Geometry check sheet. Reference: drawing and pictorial views, mm from the part's lowest x, y, z. Round coordinates to 2 decimals unless told otherwise and drop trailing zeros. Order: outer loops, then holes, each group sorted by start corner. A loop starts at its lowest first (then second) coordinate and runs counter-clockwise, first axis right, second up. Notation, with made-up numbers: (69, -29) -> (79, -29) arc R18 cw to (79, -16) -> close; hole circle Ø5 at (-9, -27). An arc over 180 degrees is marked (long way). Return JSON: item names as keys, results as strings. Group by question number.
1) Scan lines: L1, parallel to X at y = 1, z = 47; L2, parallel to Z at x = 88.5, y = 0.6; L3, parallel to Z at x = 115, y = 0.7. Record each from-to range of solid material in increasing order.
2) Section check A-A on x = 8. Enter the section's corners in (y, z), plus the area to 3 significant figures.
3) Section check C-C on y = 1.65. Enter the section's corners in (x, z).
4) Section check B-B on z = 43. Enter the section's corners in (x, y), plus the area to 3 significant figures.
5) Draft check along Y on the marked faces 1 and 2. Enter one of: pulls with the +Y half, pulls with the -Y half, needs draft (parallel to the pull), parting line crosses it, or undercut.
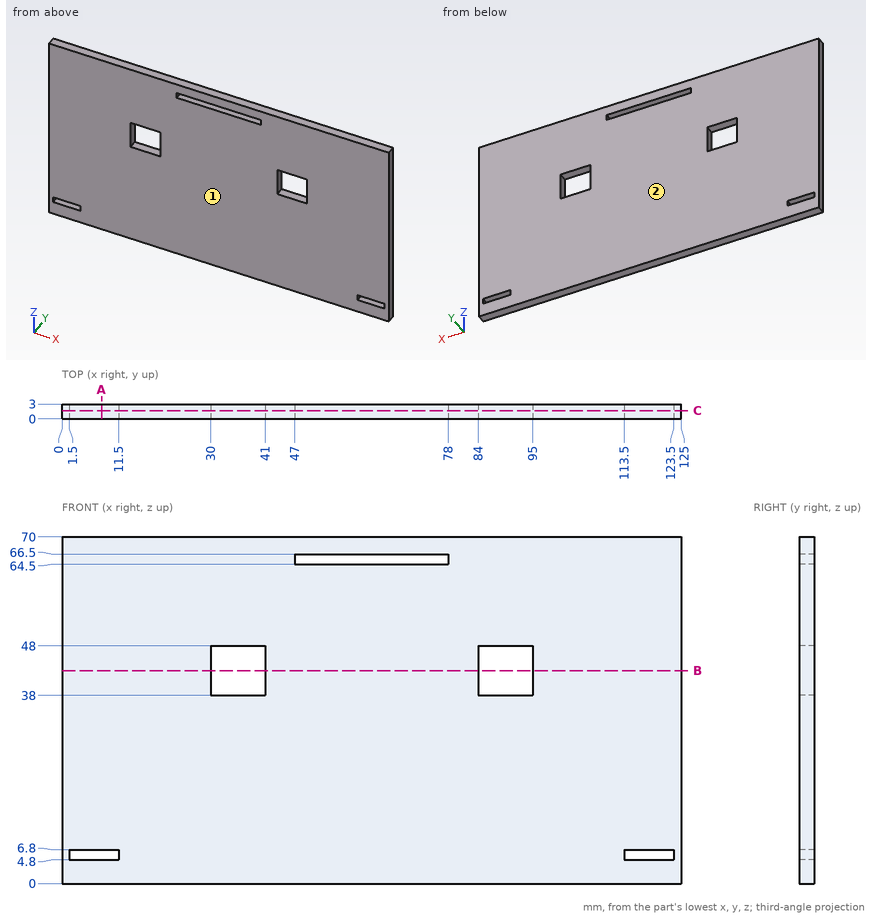
Check result:
{
 "1": {"L1": "0 to 30, 41 to 84, 95 to 125", "L2": "0 to 38, 48 to 70", "L3": "0 to 4.8, 6.8 to 70"},
 "2": {"outline": "(0, 0) -> (3, 0) -> (3, 4.8) -> (0, 4.8) -> close; (0, 6.8) -> (3, 6.8) -> (3, 70) -> (0, 70) -> close", "area": "204 mm^2"},
 "3": {"outline": "(0, 0) -> (125, 0) -> (125, 70) -> (0, 70) -> close; hole (1.5, 4.8) -> (11.5, 4.8) -> (11.5, 6.8) -> (1.5, 6.8) -> close; hole (30, 38) -> (41, 38) -> (41, 48) -> (30, 48) -> close; hole (47, 64.5) -> (78, 64.5) -> (78, 66.5) -> (47, 66.5) -> close; hole (84, 38) -> (95, 38) -> (95, 48) -> (84, 48) -> close; hole (113.5, 4.8) -> (123.5, 4.8) -> (123.5, 6.8) -> (113.5, 6.8) -> close"},
 "4": {"outline": "(0, 0) -> (30, 0) -> (30, 3) -> (0, 3) -> close; (41, 0) -> (84, 0) -> (84, 3) -> (41, 3) -> close; (95, 0) -> (125, 0) -> (125, 3) -> (95, 3) -> close", "area": "309 mm^2"},
 "5": {"face 1": "pulls with the -Y half", "face 2": "pulls with the +Y half"}
}
